The model under review builds one solid part; all positions refer to its coordinate system, in mm. A direction names the side the tool comes from. Give positions to 0.01 mm unless a question says otherwise; leave off trailing zeros. Order: outer loops, then holes, each group sorted by start corner. A loop starts at its lowest first (then second) coordinate and runs counter-clockwise, first axis right, second up. Notation, with made-up numbers: (-5, -32.5) - (46, -32.5) arc R14 ccw to (46, -7.5) - close; hole circle Ø10 at (45.5, 18). An arc over 180 degrees is marked (long way). Put each result on its own line as item: value.
Autodesk Inventor part; units mm, degrees
ref_plane "YZ Plane" through (0, 0, 0) normal (1, 0, 0) x (0, 1, 0)
ref_plane "XZ Plane" through (0, 0, 0) normal (0, 1, 0) x (-1, 0, 0)
ref_plane "XY Plane" through (0, 0, 0) normal (0, 0, 1) x (1, 0, 0)
sketch "Sketch1" plane through (0, 0, 0) normal (0, 0, 1) x (1, 0, 0)
  line L0 (0, 0) -> (76.2, 0)
  line L1 (76.2, 0) -> (76.2, 125.8)
  line L2 (76.2, 125.8) -> (0, 125.8)
  line L3 (0, 125.8) -> (0, 0)
  circle A0 centre (12, 62.9) radius 4
  circle A1 centre (42, 62.9) radius 4
  dimension "d0" = 76.2
  dimension "d1" = 125.8
  dimension "d2" = 8
  dimension "d3" = 8
  dimension "d4" = 12
  dimension "d5" = 42
  dimension "d6" = 62.9
  dimension "d7" = 62.9
extrude "Extrusion1" add sketch "Sketch1" along normal blind 38.2 contours L3 L2 L1 L0 | A0 | A1
sketch "Sketch2" plane through (0, 0, 38.2) normal (0, 0, 1) x (1, 0, 0)
  line L0 (0, 0) -> (76.2, 0)
  line L1 (76.2, 0) -> (76.2, 125.8)
  line L2 (76.2, 125.8) -> (0, 125.8)
  line L3 (0, 125.8) -> (0, 0)
  circle A0 centre (12, 62.9) radius 4
  circle A1 centre (42, 62.9) radius 4
  dimension "d17" = 76.2
  dimension "d16" = 125.8
  dimension "d13" = 8
  dimension "d10" = 8
  dimension "d15" = 12
  dimension "d12" = 42
  dimension "d11" = 62.9
  dimension "d14" = 62.9
extrude "Extrusion2" cut sketch "Sketch2" against normal blind 19.1 contours A0 | A1
sketch "Sketch3" plane through (0, 0, 0) normal (-1, 0, 0) x (0, 0, 1)
  circle A0 centre (19.1, 62.9) radius 8
  line L0 (38.2, 125.8) -> (38.2, 0)
  line L1 (0, 0) -> (38.2, 0)
  dimension "d21" = 16
  dimension "d22" = 19.1
  dimension "d23" = 62.9
extrude "Extrusion3" cut sketch "Sketch3" against normal up to next
thread "Thread1"
thread "Thread2"
sketch "Sketch7" plane through (76.2, 107.525, 0) normal (0, 0, -1) x (-1, 0, 0)
  circle A0 centre (6.335, -95.665) radius 2.5
  circle A1 centre (6.335, 6.335) radius 2.5
  line L0 (0, -89.33) -> (76.2, -89.33)
  line L1 (0, -107.525) -> (0, 18.275)
  line L2 (0, 18.275) -> (76.2, 18.275)
  point P0 (76.2, -107.525)
  dimension "d92" = 5
  dimension "d93" = 5
  dimension "d104" = 102
  dimension "d129" = 6.335
  dimension "d130" = 11.94
  dimension "d131" = 6.335
extrude "Extrusion7" cut sketch "Sketch7" against normal up to next
thread "Thread11"
thread "Thread12"
sketch "Sketch8" plane through (0, 0, 0) normal (0, 0, -1) x (-1, 0, 0)
  circle A0 centre (-8, 45.485) radius 4
  circle A1 centre (-8, 80.235) radius 4
  circle A2 centre (-68.2, 45.485) radius 4
  circle A3 centre (-68.2, 80.235) radius 4
  line L0 (0, 125.8) -> (0, 0)
  line L1 (-76.2, 0) -> (-76.2, 125.8)
  line L2 (-76.2, 18.195) -> (0, 18.195)
  line L3 (0, 107.525) -> (-76.2, 107.525)
  dimension "d106" = 8
  dimension "d107" = 8
  dimension "d108" = 8
  dimension "d109" = 8
  dimension "d110" = 8
  dimension "d111" = 8
  dimension "d112" = 8
  dimension "d113" = 8
  dimension "d114" = 34.75
  dimension "d115" = 34.75
  dimension "d116" = 27.29
  dimension "d117" = 27.29
  dimension "d118" = 89.33
extrude "Extrusion8" cut sketch "Sketch8" against normal blind 20 contours A0 | A1 | A2 | A3
thread "Thread13"
thread "Thread14"
thread "Thread15"
thread "Thread16"
sketch "Sketch9" plane through (0, 0, 0) normal (0, 0, -1) x (-1, 0, 0)
  circle A0 centre (-69.865, 113.86) radius 10
  circle A1 centre (-69.865, 11.86) radius 10
  circle A2 centre (-69.865, 113.86) radius 2.5
  circle A3 centre (-69.865, 11.86) radius 2.5
  point P0 (0, 0)
  dimension "d132" = 20
  dimension "d133" = 20
extrude "Extrusion9" cut sketch "Sketch9" against normal blind 12.67
chamfer "Chamfer2" distance 2 angle 45 4 edges at (76.2, 106.1226, 6.335) (76.2, 121.5974, 6.335) (76.2, 4.1226, 6.335) (76.2, 19.5974, 6.335)
properties part number "MotorMountLeft" material "Aluminum 6061"
(1) Take a section at D-D, the plane y = 11.86. Write out the cut boundary in (x, z) (3 decimals), then the cut area to 3 significant figures.
The answers:
outline: (0, 0) - (59.865, 0) - (59.865, 12.67) - (67.365, 12.67) - (67.365, 38.2) - (0, 38.2) - close; (72.365, 12.67) - (76.2, 12.67) - (76.2, 38.2) - (72.365, 38.2) - close
area: 2,580 mm^2
(2) Take a section at B-B, the plane z = 15. Write out the cut boundary in (x, y) (1 decimal).
The answers:
outline: (0, 0) - (76.2, 0) - (76.2, 56) - (0, 56) - close; (0, 69.8) - (76.2, 69.8) - (76.2, 125.8) - (0, 125.8) - close; hole circle Ø8 at (8, 45.5); hole circle Ø8 at (8, 80.2); hole circle Ø8 at (68.2, 45.5); hole circle Ø8 at (68.2, 80.2); hole circle Ø5 at (69.9, 11.9); hole circle Ø5 at (69.9, 113.9)
(3) The part is to be moulded in two halves that separate along Y. For faces 1 (the flat face through (38, 0, 19)), 2 (the cylindrical face through (8, 63, 32)), 3 (the cylindrical face through (8.52, 84.2, 9.86)), 4 (the flat face through (37.6, 63.8, 38.2)), say which applies: pulls with the +Y half, pulls with the -Y half, needs draft (parallel to the pull), parting line crosses it, or undercut.
The answers:
face 1: pulls with the -Y half
face 2: undercut
face 3: undercut
face 4: needs draft
(4) Clearance check with flat-ended pins moving along their axes: pin 1 Ø5 at (x, y) = (8, 45.485) entering from -Z; pin 2 Ø6.5 at (x, y) = (42, 62.9) entering from +Z; pin 3 Ø8 at (x, y) = (72, 14) entering from -Z. State where each tip first meets the part, or that it passes through.
The answers:
pin 1: z = 20
pin 2: z = 11.79
pin 3: z = 12.67
(5) For faces 5 (the cylindrical face through (59.87, 113.57, 6.25)), 6 (the cylindrical face through (67.48, 114.61, 25.26)), 7 (the cylindrical face through (38, 63, 32)), list the 3-axis set-ups (+Z, -Z, +X, -X, +Y, -Y) from which the entire face can be reached by the end or side of a thin tool; tool diameter is ignored.
The answers:
face 5: -Z
face 6: +Z, -Z
face 7: +Z
(6) Take a section at C-C, the plane z = 22.5. Write out the cut boundary in (x, y) (3 decimals).
The answers:
outline: (0, 0) - (76.2, 0) - (76.2, 55.658) - (0, 55.658) - close; (0, 70.142) - (76.2, 70.142) - (76.2, 125.8) - (0, 125.8) - close; hole circle Ø5 at (69.865, 11.86); hole circle Ø5 at (69.865, 113.86)
(7) Take a section at A-A, the plane y = 62.9. Write out the cut boundary in (x, z).
The answers:
outline: (0, 0) - (76.2, 0) - (76.2, 11.1) - (0, 11.1) - close; (0, 27.1) - (8, 27.1) - (8, 38.2) - (0, 38.2) - close; (16, 27.1) - (38, 27.1) - (38, 38.2) - (16, 38.2) - close; (46, 27.1) - (76.2, 27.1) - (76.2, 38.2) - (46, 38.2) - close
(8) Wall thickness on L1, parallel to Y at x = 70, z = 27.5; L2, parallel to Y at x = 8, z = 7.75 (3 decimals); L3, parallel to X at y = 62, z = 32: over which ranges is each line inside the solid? List them lowest first.
The answers:
L1: 0 to 9.36, 14.36 to 111.36, 116.36 to 125.8
L2: 0 to 41.485, 49.485 to 76.235, 84.235 to 125.8
L3: 0 to 8.1, 15.9 to 38.1, 45.9 to 76.2
